Geometry check sheet. Reference: the model listing, model coordinates, mm. A direction names the side the tool comes from. Round coordinates to 2 decimals unless told otherwise and drop trailing zeros. Order: outer loops, then holes, each group sorted by start corner. A loop starts at its lowest first (then second) coordinate and runs counter-clockwise, first axis right, second up. Notation, with made-up numbers: (71.5, -28) -> (78.5, -28) arc R19 cw to (78.5, -12) -> close; hole circle Ø9 at (65, 17.25). An arc over 180 degrees is marked (long way). Use a Markdown table: item, result. Add a question column.
Item 1: Set-up check for faces 5 (the flat face through (8.5, 5, -4)), 6 (the flat face through (10, 5, -10.25)): record each of +Z, -Z, +X, -X, +Y, -Y from which the full face is reachable in a straight line by a thin tool's end or side.
Item 2: Sectioned sample at C-C, the plane z = -5.75. Record the cut outline in (x, y), and give its area (3 significant figures).
Item 3: Sectioned sample at A-A, the plane x = -4.5. Record the cut outline in (y, z).
Item 4: Sectioned sample at D-D, the plane x = -10.5. Record the cut outline in (y, z), and give its area (3 significant figures).
Item 5: Mould release check, pull along X, two halves, no side actions. Record for faces 1 (the flat face through (-8.5, 5, -4)), 2 (the flat face through (-12, 5, -4)), 3 (the flat face through (0, 5, 1.75)), 4 (the flat face through (12, 5, -4)): pulls with the +X half, pulls with the -X half, needs draft (parallel to the pull), parting line crosses it, or undercut.
Item 6: Material ranges on probe 1 along X at (y, z) = (5, 0.65); probe 2 along Y at (x, z) = (9.3, -6.25); probe 3 along X at (y, z) = (2.75, -3), recorded low to high. Write a range as [from, to].
Item 7: Sectioned sample at B-B, the plane y = 5. Record the cut outline in (x, z), and give its area (3 significant figures).
Item 8: Gauge pin test, flat ends, axial feed: pin 1 Ø5 at (y, z) = (5, -6.25) entering from +X; pin 2 Ø1.9 at (x, y) = (4.5, 5) entering from -Z; pin 3 Ø3 at (x, y) = (0.5, 6) entering from -Z. Record the tip position at first contact, or that the pin passes through.
from build123d import *

# Parameters (mm, degrees)
SKETCH1_W                                           = 17
SKETCH1_H                                           = 3.5
BOSS_EXTRUDE1_DEPTH                                 = 10
SKETCH2_R                                           = 1.6
CUT_EXTRUDE1_DEPTH                                  = 25
SKETCH3_R                                           = 1.5
CUT_EXTRUDE2_DEPTH                                  = 4.5
CSK_FOR_M4_COUNTERSUNK_FLAT_HEAD_SCREW1_D           = 3.1
CSK_FOR_M4_COUNTERSUNK_FLAT_HEAD_SCREW1_CSINK_D     = 6
CSK_FOR_M4_COUNTERSUNK_FLAT_HEAD_SCREW1_CSINK_ANGLE = 90


with BuildPart() as part:
    # Sketch1 → Boss-Extrude1 (new body)
    with BuildSketch(Plane(origin=(0, 0, 0), x_dir=(1, 0, 0), z_dir=(0, 1, 0))):
        Polygon((-12, -1.75), (-8.5, -1.75), (-8.5, 1.75), (-8.5, 10.25), (-12, 10.25), align=None)
        Rectangle(SKETCH1_W, SKETCH1_H)
        Polygon((8.5, 1.75), (8.5, -1.75), (12, -1.75), (12, 10.25), (8.5, 10.25), align=None)
    extrude(amount=BOSS_EXTRUDE1_DEPTH)

    # Sketch2 → Cut-Extrude1 (cut, through all)
    with BuildSketch(Plane.ZY.offset(12)):
        with Locations((-6.25, 5)):
            Circle(SKETCH2_R)
    extrude(amount=-CUT_EXTRUDE1_DEPTH, mode=Mode.SUBTRACT)

    # Sketch3 → Cut-Extrude2 (cut, through all)
    with BuildSketch(Plane(origin=(0, 0, -1.75), x_dir=(-1, 0, 0), z_dir=(0, 0, -1))):
        with Locations((-4.5, 5)):
            Circle(SKETCH3_R)
        with Locations((4.5, 5)):
            Circle(SKETCH3_R)
    extrude(amount=-CUT_EXTRUDE2_DEPTH, mode=Mode.SUBTRACT)

    # CSK for M4 Countersunk Flat Head Screw1 (through all)
    with Locations(Plane(origin=(4.5, 5, -1.75), x_dir=(-1, 0, 0), z_dir=(0, 0, -1))):
        with Locations((0, 0), (9, 0)):
            CounterSinkHole(CSK_FOR_M4_COUNTERSUNK_FLAT_HEAD_SCREW1_D / 2, CSK_FOR_M4_COUNTERSUNK_FLAT_HEAD_SCREW1_CSINK_D / 2, counter_sink_angle=CSK_FOR_M4_COUNTERSUNK_FLAT_HEAD_SCREW1_CSINK_ANGLE)


solid = part.part
Found:
| question | item | result |
|---|---|---|
| 1 | face 5 | -Z, +Y, -Y |
| 1 | face 6 | -Z, +X, -X, +Y, -Y |
| 2 | outline | (-12, 0) -> (-8.5, 0) -> (-8.5, 3.48) -> (-12, 3.48) -> close; (-12, 6.52) -> (-8.5, 6.52) -> (-8.5, 10) -> (-12, 10) -> close; (8.5, 0) -> (12, 0) -> (12, 3.48) -> (8.5, 3.48) -> close; (8.5, 6.52) -> (12, 6.52) -> (12, 10) -> (8.5, 10) -> close |
| 2 | area | 48.7 mm2 |
| 3 | outline | (0, -1.75) -> (2, -1.75) -> (3.45, -0.3) -> (3.45, 1.75) -> (0, 1.75) -> close; (6.55, -0.3) -> (8, -1.75) -> (10, -1.75) -> (10, 1.75) -> (6.55, 1.75) -> close |
| 4 | outline | (0, -10.25) -> (10, -10.25) -> (10, 1.75) -> (0, 1.75) -> close; hole circle Ø3.2 at (5, -6.25) |
| 4 | area | 112 mm2 |
| 5 | face 1 | undercut |
| 5 | face 2 | pulls with the -X half |
| 5 | face 3 | needs draft |
| 5 | face 4 | pulls with the +X half |
| 6 | probe 1 | x = [-12, -6.05], [-2.95, 2.95], [6.05, 12] |
| 6 | probe 2 | y = [0, 3.4], [6.6, 10] |
| 6 | probe 3 | x = [-12, -8.5], [8.5, 12] |
| 7 | outline | (-12, -10.25) -> (-8.5, -10.25) -> (-8.5, -7.85) -> (-12, -7.85) -> close; (-12, -4.65) -> (-8.5, -4.65) -> (-8.5, -1.75) -> (-7.5, -1.75) -> (-6.05, -0.3) -> (-6.05, 1.75) -> (-12, 1.75) -> close; (-2.95, -0.3) -> (-1.5, -1.75) -> (1.5, -1.75) -> (2.95, -0.3) -> (2.95, 1.75) -> (-2.95, 1.75) -> close; (6.05, -0.3) -> (7.5, -1.75) -> (8.5, -1.75) -> (8.5, -4.65) -> (12, -4.65) -> (12, 1.75) -> (6.05, 1.75) -> close; (8.5, -10.25) -> (12, -10.25) -> (12, -7.85) -> (8.5, -7.85) -> close |
| 7 | area | 95.2 mm2 |
| 8 | pin 1 | stops at x = 12 |
| 8 | pin 2 | passes through |
| 8 | pin 3 | stops at z = -1.75 |
